Read the model definition and answer for the solid it produces. Units are mm, in the model's axes. Give positions to 0.01 mm unless a question says otherwise; leave off trailing zeros. Order: outer loops, then holes, each group sorted by start corner. A loop starts at its lowest first (then second) coordinate and runs counter-clockwise, first axis right, second up.
```python
from build123d import *

# Parameters (mm, degrees)
F0_W     = 500
F0_H     = 400
F1_DEPTH = 50
F2_T     = -1
F4_W     = 500
F4_H     = 400
F5_DEPTH = 1


with BuildPart() as f1:
    # F0 (on Top) → F1 (new body)
    with BuildSketch(Plane.XY):
        Rectangle(F0_W, F0_H)
    extrude(amount=F1_DEPTH)

    # F2
    f2_openings = [f1.faces().sort_by_distance(p)[0] for p in [
        (0, 0, 50),
    ]]
    offset(amount=F2_T, openings=f2_openings)

    # F4 (on offset) → F5 (join)
    with BuildSketch(Plane.XY.offset(50)):
        Rectangle(F4_W, F4_H)
    extrude(amount=F5_DEPTH)


solid = f1.part
```
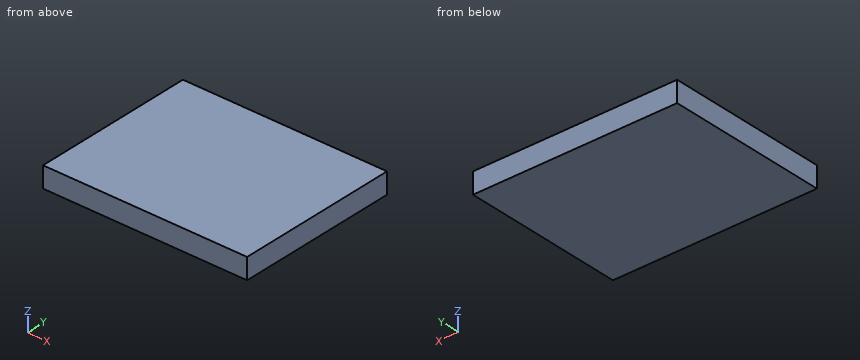
1) The part is cut by section B-B on y = 69. Determine the outline of the cut face in (x, z), and give its area (3 significant figures).
Final values:
outline: (-250, 0) - (250, 0) - (250, 51) - (-250, 51) - close; hole (-249, 1) - (249, 1) - (249, 50) - (-249, 50) - close
area: 1,100 mm2
2) Consider L1, parallel to Y at x = 143, z = 15; L2, parallel to Z at x = -153, y = -99; L3, parallel to X at y = 150, z = 7. Determine where each line is inside the solid, lowest interval first.
Final values:
L1: y = -200 to -199, 199 to 200
L2: z = 0 to 1, 50 to 51
L3: x = -250 to -249, 249 to 250
3) The part is cut by section A-A on z = 42. Determine the outline of the cut face in (x, y).
Final values:
outline: (-250, -200) - (250, -200) - (250, 200) - (-250, 200) - close; hole (-249, -199) - (249, -199) - (249, 199) - (-249, 199) - close
